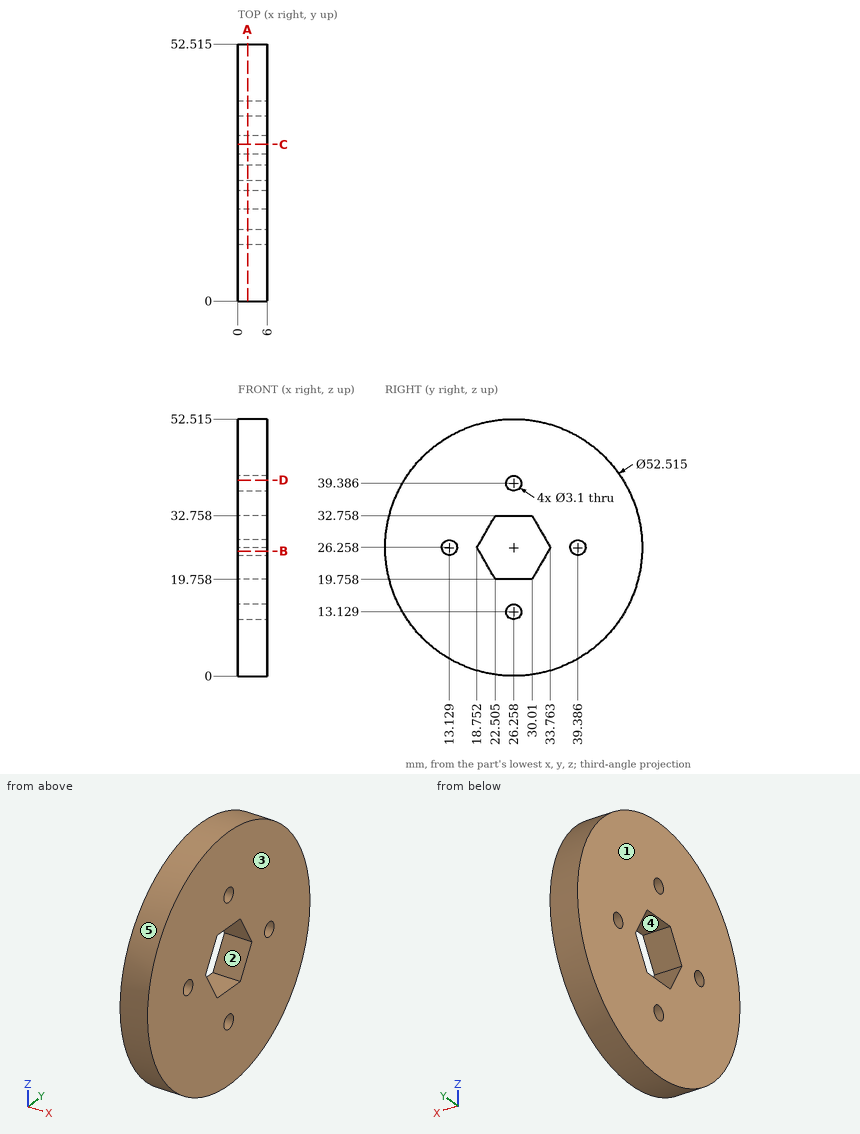
Check sheet for the drawn part. Datum: minimum x, y, z corner. Units: mm. A direction names the side the tool comes from. Round coordinates to 2 decimals unless told otherwise and drop trailing zeros. Order: outer loops, then holes, each group sorted by start corner. A loop starts at its lowest first (then second) coordinate and runs counter-clockwise, first axis right, second up.
(1) Cross-section at B-B, the plane z = 25.5. Enter the section's corners in (x, y) (1 decimal), and give its area (3 significant figures).
(2) Draft check along Z on the marked faces 3, 4 and 5. Enter one of: pulls with the +Z half, pulls with the -Z half, needs draft (parallel to the pull), parting line crosses it, or undercut.
(3) Scan lines: probe 1 along Z at (x, y) = (1.45, 27) (1 decimal); probe 2 along Y at (x, z) = (1.2, 27) (1 decimal); probe 3 along Z at (x, y) = (3.5, 39) (1 decimal). Record each from-to range of solid material in increasing order.
(4) Access from +Z, -Z, +X, -X, +Y, -Y to the whole of each face (thin tool, end or side, straight path). Record for the marked faces 1 and 2.
(5) Go/stop test with flat-tipped pins: P1, Ø3, axis at x = 3.5, z = 16, coming from the +Y side; P2, Ø2, axis at x = 4.5, z = 42, coming from the -Y side; P3, Ø1.5, axis at x = 4, y = 18, coming from the -Z side. Record where each tip stops, or that it passes through.
(6) Cross-section at C-C, the plane y = 32. Enter the section's corners in (x, z) (1 decimal).
(7) Cross-section at A-A, the plane x = 2. State how many separate pieces and enclosed holes the cut face has, and give its area (3 significant figures).
(8) Cross-section at D-D, the plane z = 40. Enter the section's corners in (x, y) (1 decimal).
Check sheet entries:
1. outline: (0, 0) - (6, 0) - (6, 11.8) - (0, 11.8) - close; (0, 14.5) - (6, 14.5) - (6, 19.2) - (0, 19.2) - close; (0, 33.3) - (6, 33.3) - (6, 38) - (0, 38) - close; (0, 40.7) - (6, 40.7) - (6, 52.5) - (0, 52.5) - close
1. area: 198 mm2
2. face 3: needs draft
2. face 4: undercut
2. face 5: parting line crosses it
3. probe 1: z = 0 to 11.8, 14.5 to 19.8, 32.8 to 38, 40.7 to 52.5
3. probe 2: y = 0 to 11.8, 14.5 to 19.2, 33.3 to 38, 40.7 to 52.5
3. probe 3: z = 3.3 to 24.8, 27.8 to 49.2
4. face 1: +Z, -Z, -X, +Y, -Y
4. face 2: +X, -X
5. P1: stops at y = 51.01
5. P2: stops at y = 4.53
5. P3: stops at z = 1.1
6. outline: (0, 0.6) - (6, 0.6) - (6, 23.2) - (0, 23.2) - close; (0, 29.3) - (6, 29.3) - (6, 51.9) - (0, 51.9) - close
7. separate pieces: 1
7. enclosed holes: 5
7. area: 1,990 mm2
8. outline: (0, 3.9) - (6, 3.9) - (6, 24.8) - (0, 24.8) - close; (0, 27.7) - (6, 27.7) - (6, 48.6) - (0, 48.6) - close
